Drawing for the job (mm, zero at the part's lowest x, y, z). A direction names the side the tool comes from. Give positions to 0.01 mm unless a question says otherwise; leave off trailing zeros. Order: outer loops, then holes, each group sorted by start corner. A loop starts at its lowest first (then second) coordinate and runs counter-clockwise, first axis right, second up. Notation, with made-up numbers: (42, 38) - (100, 38) arc R22 ccw to (100, 45) - close; hole circle Ø4 at (26.5, -0.75). An arc over 180 degrees is marked (long way). Use a Markdown table: item, result.
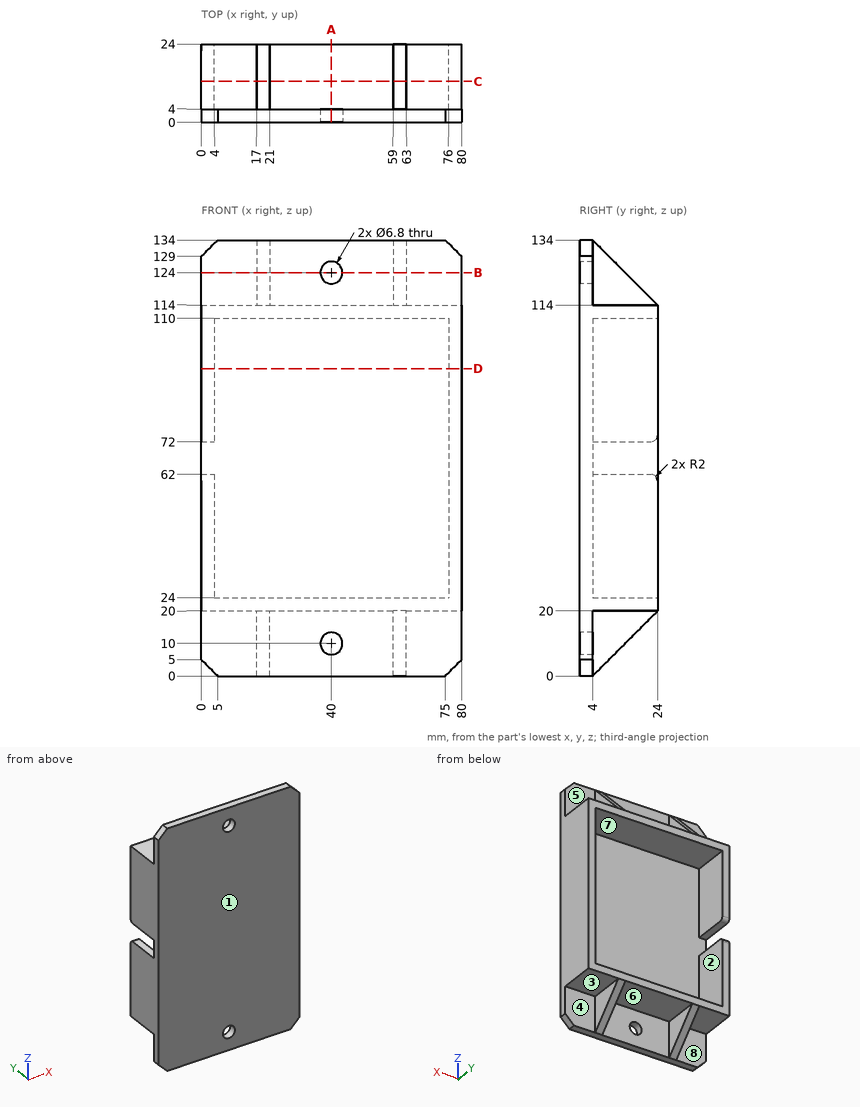
1) Tool access for the marked faces 4, 5, 6, 7 and 8: list every direction of +Z, -Z, +X, -X, +Y, -Y with a clear straight run to the whole face (end or side of a thin tool).
Computed:
| item | result |
|---|---|
| face 4 | -Z, +X, +Y |
| face 5 | +Z, +X, +Y |
| face 6 | -Z, +Y |
| face 7 | +Y |
| face 8 | -Z, -X, +Y |
2) Slice it at D-D (z = 94.5). Write the cut outline in (x, y), and give its area (3 significant figures).
Computed:
| item | result |
|---|---|
| outline | (0, 0) - (80, 0) - (80, 24) - (76, 24) - (76, 4) - (4, 4) - (4, 24) - (0, 24) - close |
| area | 480 mm² |
3) Two-plate mould, pull along Z, no slides. Class the marked faces 1, 2 and 3: +Z half, -Z half, draft (parallel to the pull), parting line (faces both ways), or undercut.
Computed:
| item | result |
|---|---|
| face 1 | draft |
| face 2 | undercut |
| face 3 | -Z half |
4) Slice it at B-B (z = 124). Write the cut outline in (x, y), and give its area (3 significant figures).
Computed:
| item | result |
|---|---|
| outline | (0, 0) - (36.6, 0) - (36.6, 4) - (21, 4) - (21, 14) - (17, 14) - (17, 4) - (0, 4) - close; (43.4, 0) - (80, 0) - (80, 4) - (63, 4) - (63, 14) - (59, 14) - (59, 4) - (43.4, 4) - close |
| area | 373 mm² |
5) Pin check, flat tips, straight feed: P1, Ø2, axis at x = 19, y = 21.5, coming from the +Z side; P2, Ø13.5, axis at x = 71.5, y = 11.5, coming from the +Z side; P3, Ø6, axis at x = 35, y = 19, coming from the -Z side; P4, Ø10, axis at y = 18.5, z = 127.5, coming from the -X side. Stop position of each tip, or through.
Computed:
| item | result |
|---|---|
| P1 | stops at z = 117.5 |
| P2 | stops at z = 114 |
| P3 | stops at z = 20 |
| P4 | passes through |
6) Slice it at A-A (x = 40). Write the cut outline in (y, z).
Computed:
| item | result |
|---|---|
| outline | (0, 0) - (4, 0) - (4, 6.6) - (0, 6.6) - close; (0, 13.4) - (4, 13.4) - (4, 20) - (24, 20) - (24, 24) - (4, 24) - (4, 110) - (24, 110) - (24, 114) - (4, 114) - (4, 120.6) - (0, 120.6) - close; (0, 127.4) - (4, 127.4) - (4, 134) - (0, 134) - close |
7) Slice it at C-C (y = 12.5). Write the cut outline in (x, z), and give its area (3 significant figures).
Computed:
| item | result |
|---|---|
| outline | (0, 20) - (17, 20) - (17, 8.5) - (21, 8.5) - (21, 20) - (59, 20) - (59, 8.5) - (63, 8.5) - (63, 20) - (80, 20) - (80, 114) - (63, 114) - (63, 125.5) - (59, 125.5) - (59, 114) - (21, 114) - (21, 125.5) - (17, 125.5) - (17, 114) - (0, 114) - (0, 72) - (4, 72) - (4, 110) - (76, 110) - (76, 24) - (4, 24) - (4, 62) - (0, 62) - close |
| area | 1,470 mm² |
8) Wall check: line 1 (X direction, y = 6.5, z = 30.5); line 2 (Z direction, x = 51.5, y = 14); line 3 (X direction, y = 1.9, z = 10). Give the ranges that are in metal, low to high. Write a range as from..to.
Computed:
| item | result |
|---|---|
| line 1 | x = 0..4, 76..80 |
| line 2 | z = 20..24, 110..114 |
| line 3 | x = 0..36.6, 43.4..80 |
